For this review, take the finished solid that the model builds, in its own axes (mm). A direction names the side the tool comes from. Give positions to 0.01 mm unless a question says otherwise; leave off trailing zeros. Write each loop counter-clockwise with the first axis right and the second up, starting at its lowest first coordinate (ties: lowest second). Pieces come first, ordered by that corner, then holes. Notation, with made-up numbers: (51.5, 68.25) -> (101.5, 68.25) arc R22 cw to (101.5, 82.25) -> close; hole circle Ø5 at (1, 24.5). An arc over 180 degrees is marked (long way). Answer as CSV lines item,"result".
```python
from build123d import *

# Parameters (mm, degrees)
SKETCH1_W           = 72
SKETCH1_H           = 42
BOSS_EXTRUDE1_DEPTH = 12
SKETCH2_W           = 40
SKETCH2_H           = 28
BOSS_EXTRUDE2_DEPTH = 28
SKETCH3_R           = 12
CUT_EXTRUDE1_DEPTH  = 29
BOSS_EXTRUDE3_DEPTH = 8
FILLET3_R           = 16
SKETCH5_R           = 6
CUT_EXTRUDE2_DEPTH  = 13


with BuildPart() as part:
    # Sketch1 → Boss-Extrude1 (new body)
    with BuildSketch(Plane(origin=(0, 0, 0), x_dir=(1, 0, 0), z_dir=(0, 1, 0))):
        Rectangle(SKETCH1_W, SKETCH1_H)
    extrude(amount=BOSS_EXTRUDE1_DEPTH)

    # Sketch2 → Boss-Extrude2 (add)
    with BuildSketch(Plane(origin=(0, 12, 0), x_dir=(1, 0, 0), z_dir=(0, 1, 0))):
        with Locations((-16, 7)):
            Rectangle(SKETCH2_W, SKETCH2_H)
    extrude(amount=BOSS_EXTRUDE2_DEPTH)

    # Sketch3 → Cut-Extrude1 (cut, through all)
    with BuildSketch(Plane.XY.offset(7)):
        with Locations((-16, 40)):
            Circle(SKETCH3_R)
    extrude(amount=-CUT_EXTRUDE1_DEPTH, mode=Mode.SUBTRACT)

    # Sketch4 → Boss-Extrude3 (add)
    with BuildSketch(Plane(origin=(0, 0, -21), x_dir=(-1, 0, 0), z_dir=(0, 0, -1))):
        Polygon((-4, 40), (-4, 12), (-36, 12), align=None)
    extrude(amount=-BOSS_EXTRUDE3_DEPTH)

    # Fillet3
    fillet3_edges = [part.edges().sort_by_distance(p)[0] for p in [
        (36, 6, 21),
    ]]
    fillet(fillet3_edges, radius=FILLET3_R)

    # Sketch5 → Cut-Extrude2 (cut, through all)
    with BuildSketch(Plane(origin=(0, 12, 0), x_dir=(1, 0, 0), z_dir=(0, 1, 0))):
        with Locations((20, -5)):
            Circle(SKETCH5_R)
    extrude(amount=-CUT_EXTRUDE2_DEPTH, mode=Mode.SUBTRACT)


solid = part.part
```
Q1. Add section C-C (x = 2). Write out the cut boundary in (y, z).
Answer block:
outline,"(0, -21) -> (40, -21) -> (40, 7) -> (12, 7) -> (12, 21) -> (0, 21) -> close"
Q2. Draft analysis for pull direction X (two halves, no side actions). For faces 1 (the cylindrical face through (25.54, 6.08, 7.3)), 2 (the flat face through (4, 26, -3)), 3 (the flat face through (-16, 23, 7)), state which applies: released by +X, released by -X, zero draft, split by the parting line, or undercut.
Answer block:
face 1,"undercut"
face 2,"released by +X"
face 3,"zero draft"
Q3. For faces 4 (the flat face through (13, 20, -13)), 5 (the flat face through (-1, 0, 0)), list the 3-axis set-ups (+Z, -Z, +X, -X, +Y, -Y) from which the entire face can be reached by the end or side of a thin tool; tool diameter is ignored.
Answer block:
face 4,"+Z, +X, +Y"
face 5,"+Z, -Z, +X, -X, -Y"
Q4. Add section A-A (z = -18). Write out the cut boundary in (x, y).
Answer block:
outline,"(-36, 0) -> (36, 0) -> (36, 12) -> (4, 40) -> (-4, 40) arc R12 cw to (-28, 40) -> (-36, 40) -> close"
Q5. Add section D-D (z = 9). Write out the cut boundary in (x, y).
Answer block:
outline,"(-36, 0) -> (15.53, 0) -> (15.53, 12) -> (-36, 12) -> close; (24.47, 0) -> (35.49, 0) -> (35.49, 12) -> (24.47, 12) -> close"
Q6. Add section B-B (y = 22.5). Write out the cut boundary in (x, z), plus the area to 3 significant figures.
Answer block:
outline,"(-36, -21) -> (24, -21) -> (24, -13) -> (4, -13) -> (4, 7) -> (-36, 7) -> close"
area,"1,280 mm2"
Q7. Clearance check with flat-ended pins moving along their axes: pin 1 (10 mm diameter, centred on y = 21, z = -4.5, fed in from +X); pin 2 (1.5 mm diameter, centred on y = 12.5, z = 13, fed in from +X); pin 3 (6 mm diameter, centred on x = -16, y = 17.5, fed in from +Z); pin 4 (4 mm diameter, centred on x = 15.5, z = 16, fed in from -Y). State where each tip first meets the part, or that it passes through.
Answer block:
pin 1,"stops at x = 4"
pin 2,"stops at x = 34.16"
pin 3,"stops at z = 7"
pin 4,"stops at y = 0"
Q8. To check wall thickness, follow probe 1 along Y at (x, z) = (27, 18.5); probe 2 along X at (y, z) = (18.5, -3); probe 3 along Z at (x, y) = (13, 27). State the ranges of each line that lie inside material, in increasing order. Write a range as [from, to].
Answer block:
probe 1,"y = [0, 12]"
probe 2,"x = [-36, 4]"
probe 3,"z = [-21, -13]"
